from build123d import *

# Parameters (mm, degrees)
BOSS_EXTRUDE3_DEPTH      = 2.2
CHAMFER2_SIZE            = 0.6
CHAMFER2_SIZE_2          = 2.822778066
FILLET1_R                = 0.4
BOSS_EXTRUDE4_DEPTH      = 4.6
BOSS_EXTRUDE4_DEPTH_BACK = 1.4
SKETCH2_R                = 0.965366887
FILLET2_R                = 1.2


with BuildPart() as part:
    # Sketch1 → Boss-Extrude3 (new body)
    with BuildSketch(Plane(origin=(0, 0, 0), x_dir=(1, 0, 0), z_dir=(0, 1, 0))):
        Polygon((5.086064398, 0.292080247), (4.289535013, 2.000243026), (0, 0), (0, -4.2), (0.684040287, -6.079385242), (2.563425528, -5.395344955), (1.63771199, -2.851967912), (2.624045016, -0.142040197), align=None)
    extrude(amount=BOSS_EXTRUDE3_DEPTH)

    # Chamfer2
    # the kernel refuses this chamfer: 2.822778066, 0.6 mm, written as the material it takes off along each edge
    with BuildSketch(Plane(origin=(2.563425528, -7.333289373, 5.395344955), x_dir=(-0.865629936296976, 0, 0.5006843450583344), z_dir=(0, 1, 0))) as chamfer2_piece_1_section:
        Polygon((CHAMFER2_SIZE * 0.984670194927, -CHAMFER2_SIZE * 0.174426509515), (-CHAMFER2_SIZE_2 * 0.174426509496, -CHAMFER2_SIZE_2 * 0.984670194818), (0, 0), align=None)
    chamfer2_piece_1 = extrude(amount=16.866578746, mode=Mode.PRIVATE)
    chamfer2_piece_1 = split(chamfer2_piece_1, bisect_by=Plane(origin=(1.145577622, 1.1, 4.204095975), z_dir=(0.93969262078591, 0, 0.3420201433256644)), keep=Keep.TOP, mode=Mode.PRIVATE)
    add(chamfer2_piece_1, mode=Mode.SUBTRACT)

    # Fillet1
    fillet1_edges = [part.edges().sort_by_distance(p)[0] for p in [
        (4.289535013, 1.1, -2.000243026),
        (5.086064398, 1.1, -0.292080247),
        (2.624045016, 1.1, 0.142040197),
        (0.684040287, 1.1, 6.079385242),
        (0, 1.1, 4.2),
        (1.999609956, 1.1, 5.600557041),
        (1.620115519, 1.1, 2.900313819),
    ]]
    fillet(fillet1_edges, radius=FILLET1_R)

    # Sketch2 → Boss-Extrude4 (add, two sides: drawn at the far end of the back side and taken through both)
    with BuildSketch(Plane(origin=(0, 0, 0), x_dir=(1, 0, 0), z_dir=(0, 1, 0)).offset(-BOSS_EXTRUDE4_DEPTH_BACK)):
        with Locations(Location((1.165366887, -0.742420587, 0), (0, 0, 270))):
            Circle(SKETCH2_R)
    extrude(amount=BOSS_EXTRUDE4_DEPTH + BOSS_EXTRUDE4_DEPTH_BACK)

    # Fillet2
    fillet2_edges = [part.edges().sort_by_distance(p)[0] for p in [
        (0, 1.1, 0),
    ]]
    fillet(fillet2_edges, radius=FILLET2_R)


solid = part.part
Geometry: final body of the model. Coordinates: model frame, mm. A direction names the side the tool comes from. Give positions to 0.01 mm unless a question says otherwise; leave off trailing zeros. Order: outer loops, then holes, each group sorted by start corner. A loop starts at its lowest first (then second) coordinate and runs counter-clockwise, first axis right, second up. Notation, with made-up numbers: (37.5, 20) - (74.5, 20) arc R8 cw to (74.5, 33) - close; hole circle Ø4 at (-16, 11.5). An arc over 180 degrees is marked (long way). Use CSV: the item, a comma, the result in double quotes.
1. Material intervals for line 1 along Y through (x, z) = (1.6, 3.5); line 2 along X through (y, z) = (1.15, 2.75); line 3 along X through (y, z) = (-1.1, 0.5), sorted ascending. Write a range as from..to.
Answers below:
line 1,"0..2.2"
line 2,"0..1.67"
line 3,"0.23..2.1"
2. Section query D-D (z = -1.5). Output: boundary loops of the cut face in (x, y).
Answers below:
outline,"(3.22, 0) - (4.52, 0) - (4.52, 2.2) - (3.22, 2.2) - close"
3. Access query for faces 1 (the face through (0.31, -0.71, 1.19)), 2 (the face through (2.093, 1.085, 1.6)), 3 (the face through (3.7, 1.085, -0.048)), 4 (the face through (0.31, 3.38, 1.19)), 5 (the face through (4.665, 1.085, -1.195)). Directions: +Z, -Z, +X, -X, +Y, -Y. A direction counts if a zero-diameter tool reaches every point of the face in a straight line with its end or side. Return the directions, or none.
Answers below:
face 1,"-Y"
face 2,"+X, +Y, -Y"
face 3,"+Z, +X, +Y, -Y"
face 4,"+Y"
face 5,"-Z, +X, +Y, -Y"
4. Section query C-C (x = 4.1). Output: boundary loops of the cut face in (y, z).
Answers below:
outline,"(0, -1.87) - (2.2, -1.87) - (2.2, -0.12) - (0, -0.12) - close"
5. Section query B-B (y = -0.15). Output: boundary loops of the cut face in (x, z), plus the area to 3 significant figures.
Answers below:
outline,"circle Ø1.93 at (1.17, 0.74)"
area,"2.93 mm2"
6. Section query A-A (z = 0). Output: boundary loops of the cut face in (x, y).
Answers below:
outline,"(0.28, 0) - (0.55, 0) - (0.55, -1.4) - (1.78, -1.4) - (1.78, 0) - (3.43, 0) - (3.43, 2.2) - (1.78, 2.2) - (1.78, 4.6) - (0.55, 4.6) - (0.55, 2.2) - (0.28, 2.2) - close"
7. Contact query for a flat-ended pin moving along its axis: pin 1 (2 mm diameter, centred on x = 1.5, z = 5, fed in from -Y). Output: stop coordinate, or through.
Answers below:
pin 1,"y = 0"
